Check sheet for the modelled part. Datum: model origin and axes. Units: mm. A direction names the side the tool comes from. Give positions to 0.01 mm unless a question says otherwise; leave off trailing zeros. Loops run counter-clockwise (first coordinate to the right, second up) from the corner with the lowest first, then second, coordinate; pieces in that order, holes last. Notation, with made-up numbers: M 55.25,73 L 72.25,73 A7 ccw 72.25,84 Z; hole C 46,31 d4. An arc over 180 degrees is marked long. One line per question, with ' | ' between items. Start each with the question number.
from build123d import *

# Parameters (mm, degrees)
SKETCH_1_W          = 36
SKETCH_1_H          = 37.5
EXTRUDE_1_DEPTH     = 11.5
SKETCH_2_W          = 20
SKETCH_2_H          = 20
EXTRUDE_2_DEPTH     = 1
SKETCH_3_R          = 7
EXTRUDE_3_DEPTH     = 5
FILLET_1_R          = 0.5
SKETCH_4_R          = 4.5
CUT_EXTRUDE_1_DEPTH = 0.5


with BuildPart() as part:
    # 草图1 → 凸台-拉伸1 (new body)
    with BuildSketch(Plane.XY):
        Rectangle(SKETCH_1_W, SKETCH_1_H)
    extrude(amount=EXTRUDE_1_DEPTH)

    # 草图2 → 凸台-拉伸2 (add)
    with BuildSketch(Plane.XY.offset(11.5)):
        Rectangle(SKETCH_2_W, SKETCH_2_H)
    extrude(amount=EXTRUDE_2_DEPTH)

    # 草图3 → 凸台-拉伸3 (add)
    with BuildSketch(Plane.XY.offset(12.5)):
        Circle(SKETCH_3_R)
    extrude(amount=EXTRUDE_3_DEPTH)

    # 圆角1
    fillet_1_edges = [part.edges().sort_by_distance(p)[0] for p in [
        (18, 0, 11.5),
        (0, 18.75, 11.5),
        (-10, 0, 11.5),
        (0, -10, 11.5),
        (10, 0, 11.5),
        (0, 10, 11.5),
        (-7, 0, 17.5),
        (-18, 0, 11.5),
        (0, 18.75, 0),
        (18, 0, 0),
        (0, -18.75, 0),
        (-18, 0, 0),
        (0, -18.75, 11.5),
        (-18, 18.75, 5.75),
        (18, 18.75, 5.75),
        (18, -18.75, 5.75),
        (-18, -18.75, 5.75),
    ]]
    fillet(fillet_1_edges, radius=FILLET_1_R)

    # 草图4 → 切除-拉伸1 (cut)
    with BuildSketch(Plane.XY.offset(17.5)):
        Circle(SKETCH_4_R)
    extrude(amount=-CUT_EXTRUDE_1_DEPTH, mode=Mode.SUBTRACT)

    # 草图6 → M2 螺纹孔1 (revolve, cut)
    with BuildSketch(Plane(origin=(0, -18.75, 5.75), x_dir=(0, 0, -1), z_dir=(1, 0, 0))):
        Polygon((0, 0), (0, 20.480688495), (0.8, 20), (0.8, 0), align=None)
    hole_wizard_m2_1 = revolve(axis=Axis((0, -25.1, 5.75), (0, 1, 0)), mode=Mode.SUBTRACT)

    # 镜向1: M2 螺纹孔1 across plane
    add(hole_wizard_m2_1.mirror(Plane.ZX), mode=Mode.SUBTRACT)


solid = part.part
Q1. Cross-section at B-B (z = 5.75). Record the cut outline in (x, y), and give its area (3 significant figures).
Q2. Draft check along Y on faces 3 (the flat face through (-0.2, 18.75, 4.5)), 4 (the flat face through (0, 0, 0)), 5 (the cylindrical face through (-0.59, 4.46, 17.25)). Enter one of: released by +Y, released by -Y, zero draft, split by the parting line, or undercut.
Q3. Cross-section at C-C (y = 0). Record the cut outline in (x, z), and give its area (3 significant figures).
Q4. Access from +Z, -Z, +X, -X, +Y, -Y to the whole of each face (thin tool, end or side, straight path). Record for faces 1 (the flat face through (0, 0, 17)), 2 (the flat face through (18, 0, 6)).
Q5. Cross-section at A-A (y = 8.5). Record the cut outline in (x, z).
Q6. Depth check by flat-ended pin: P1, Ø10.5, axis at x = 6.5, y = -7.5, coming from the +Z side; P2, Ø1.5, axis at x = -9.5, y = 3.5, coming from the +Z side; P3, Ø1.3, axis at x = 0, z = 5.75, coming from the -Y side; P4, Ø2.5, axis at x = 0.5, y = -1.5, coming from the +Z side. Enter the tip coordinate at first touch or a pass-through.
Q7. Material ranges on probe 1 along Z at (x, y) = (0, 15); probe 2 along X at (y, z) = (6.5, 5.75); probe 3 along Z at (x, y) = (0, -9.75), recorded low to high. Write a range as from..to.
Solved:
1) outline: M -18,-18.25 A0.5 ccw -17.5,-18.75 L -0.8,-18.75 L -0.8,18.75 L -17.5,18.75 A0.5 ccw -18,18.25 Z; M 0.8,-18.75 L 17.5,-18.75 A0.5 ccw 18,-18.25 L 18,18.25 A0.5 ccw 17.5,18.75 L 0.8,18.75 Z | area: 1,290 mm²
2) face 3: released by +Y | face 4: zero draft | face 5: undercut
3) outline: M -18,0.5 A0.5 ccw -17.5,0 L 17.5,0 A0.5 ccw 18,0.5 L 18,11 A0.5 ccw 17.5,11.5 L 10.5,11.5 A0.5 cw 10,12 L 10,12.5 L 7,12.5 L 7,17 A0.5 ccw 6.5,17.5 L 4.5,17.5 L 4.5,17 L -4.5,17 L -4.5,17.5 L -6.5,17.5 A0.5 ccw -7,17 L -7,12.5 L -10,12.5 L -10,12 A0.5 cw -10.5,11.5 L -17.5,11.5 A0.5 ccw -18,11 Z; hole C 0,5.75 d1.6 | area: 497 mm²
4) face 1: +Z | face 2: +Z, -Z, +X, +Y, -Y
5) outline: M -18,0.5 A0.5 ccw -17.5,0 L 17.5,0 A0.5 ccw 18,0.5 L 18,11 A0.5 ccw 17.5,11.5 L 10.5,11.5 A0.5 cw 10,12 L 10,12.5 L -10,12.5 L -10,12 A0.5 cw -10.5,11.5 L -17.5,11.5 A0.5 ccw -18,11 Z; hole C 0,5.75 d1.6
6) P1: stops at z = 17.5 | P2: stops at z = 12.5 | P3: passes through | P4: stops at z = 17
7) probe 1: z = 0..4.95, 6.55..11.5 | probe 2: x = -18..-0.8, 0.8..18 | probe 3: z = 0..4.95, 6.55..12.5
